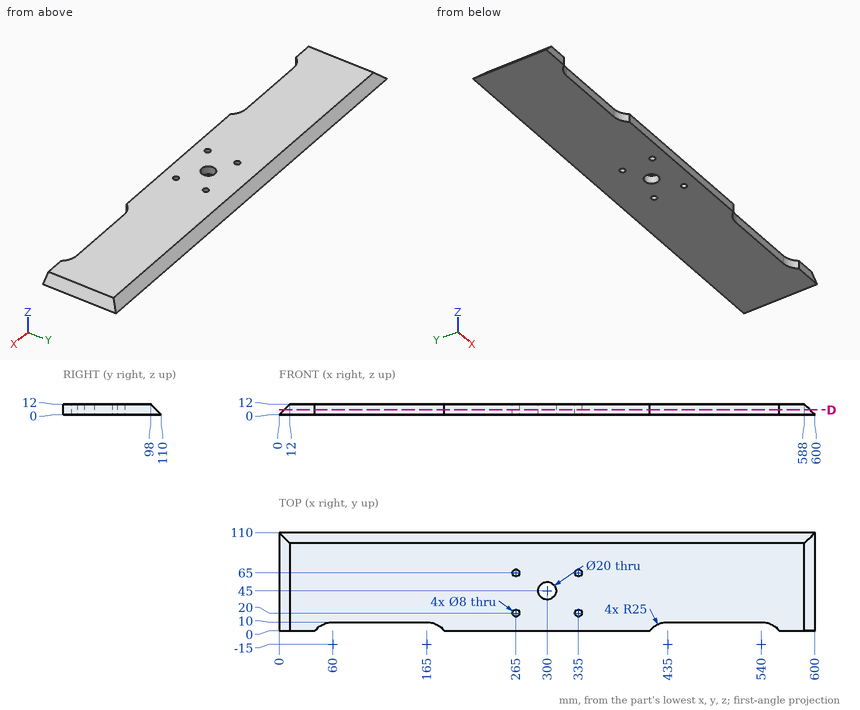
Geometry check sheet. Reference: drawing and pictorial views, mm from the part's lowest x, y, z. Coordinates: 2 decimals unless noted, no trailing zeros. Write each loop counter-clockwise with the first axis right and the second up, starting at its lowest first coordinate (ties: lowest second). Pieces come first, ordered by that corner, then holes. Notation, with made-up numbers: M 50.25,-38.75 L 91.25,-38.75 A19 cw 91.25,-18.75 Z; hole C -32,-2.75 d11. An arc over 180 degrees is marked long. Write item = value, one per line. Start each with the question number.
1. Thickness scan on probe 1 along Y at (x, z) = (335, 4); probe 2 along X at (y, z) = (62, 3.5); probe 3 along Y at (x, z) = (265, 8). Record the ranges inside material, lowest first.
2. Go/stop test with flat-tipped pins: pin 1 (1.5 mm diameter, centred on y = 94, z = 9.5, fed in from +X); pin 2 (6 mm diameter, centred on y = 23.5, z = 10, fed in from +X); pin 3 (6 mm diameter, centred on y = 29, z = 10.5, fed in from -X). Record where each tip stops, or that it passes through.
3. Sectioned sample at D-D (z = 5.5). Record the cut outline in (x, y), then the cut area to 3 significant figures.
The answers:
q1.probe_1 = 0 to 16, 24 to 61, 69 to 106
q1.probe_2 = 3.5 to 262.35, 267.65 to 332.35, 337.65 to 596.5
q1.probe_3 = 0 to 16, 24 to 61, 69 to 102
q2.pin_1 = 591.25
q2.pin_2 = 593
q2.pin_3 = 7.5
q3.outline = M 5.5,0 L 40,0 A25 cw 60,10 L 165,10 A25 cw 185,0 L 415,0 A25 cw 435,10 L 540,10 A25 cw 560,0 L 594.5,0 L 594.5,104.5 L 5.5,104.5 Z; hole C 265,20 d8; hole C 265,65 d8; hole C 300,45 d20; hole C 335,20 d8; hole C 335,65 d8
q3.area = 58,400 mm²
